Autodesk Fusion 360 part; units mm, degrees
sketch "Sketch1" plane through (0, 0, 0) normal (0, 0, 1) x (1, 0, 0)
  line L0 (0, 0) -> (-178, 0)
  line L1 (-178, 0) -> (-178, 64)
  line L2 (-178, 64) -> (0, 64)
  line L3 (0, 64) -> (0, 0)
  dimension "d1" = 64
  dimension "d2" = 178
extrude "Extrude1" add sketch "Sketch1" along normal blind 19
fillet "Fillet1" radius 32 4 edges at (0, 0, 9.5) (0, 64, 9.5) (-178, 0, 9.5) (-178, 64, 9.5)
sketch "Sketch2" plane through (0, 0, 19) normal (0, 0, 1) x (-1, 0, 0)
  arc A0 (146, -64) -> (146, 0) centre (146, -32) ccw
  line L0 (146, 0) -> (32, 0)
  arc A1 (32, 0) -> (32, -64) centre (32, -32) ccw
  line L1 (32, -64) -> (146, -64)
  line L2 (89, -64) -> (89, 0) construction
  circle A2 centre (32, -32) radius 10.5
  circle A3 centre (146, -32) radius 10.5
  dimension "d6" = 21
extrude "Extrude2" cut sketch "Sketch2" against normal blind 90 contours A2 | A3
sketch "Sketch3" plane through (0, 0, 19) normal (0, 0, 1) x (-1, 0, 0)
  circle A0 centre (32, -32) radius 10.5
  circle A1 centre (146, -32) radius 10.5
  arc A2 (146, -64) -> (146, 0) centre (146, -32) ccw
  line L0 (146, 0) -> (32, 0)
  arc A3 (32, 0) -> (32, -64) centre (32, -32) ccw
  line L1 (32, -64) -> (146, -64)
  line L2 (146, -64) -> (32, -64) construction
  line L3 (89, -64) -> (89, 0) construction
  line L4 (89, -64) -> (57, -64)
  line L5 (121, -64) -> (108, -64)
  line L6 (108, -64) -> (108, 0)
  line L7 (108, 0) -> (121, 0)
  line L8 (121, 0) -> (121, -64)
  line L9 (121, -64) -> (108, -64)
  line L10 (108, -64) -> (108, 0)
  line L11 (108, 0) -> (121, 0)
  line L12 (121, 0) -> (121, -64)
  line L13 (70, -64) -> (70, 0)
  line L14 (57, -64) -> (70, -64)
  line L15 (57, 0) -> (57, -64)
  line L16 (70, 0) -> (57, 0)
  line L17 (108, -64) -> (70, -64)
  line L18 (70, -64) -> (70, -51)
  line L19 (70, -51) -> (108, -51)
  line L20 (108, -51) -> (108, -64)
  dimension "d9" = 32
  dimension "d10" = 32
  dimension "d11" = 13
  dimension "d12" = 64
  dimension "d13" = 13
extrude "Extrude3" add sketch "Sketch3" along normal blind 45 contours L0 L1 L5 L6 L7 L8 L9 L10 L11 L12 L20 | L1 L4 L6 L10 L13 L17 L18 L19 L20 | L0 L1 L4 L13 L14 L15 L16 L18
sketch "Sketch4" plane through (-108, 0, 0) normal (1, 0, 0) x (0, 1, 0)
  line L0 (0, 19) -> (51, 19)
  line L1 (51, 19) -> (51, 64)
  line L2 (51, 64) -> (0, 64)
  line L3 (0, 64) -> (0, 19)
  line L4 (51, 64) -> (0, 19)
  line L5 (51, 19) -> (51, 64)
  line L6 (51, 19) -> (0, 19)
extrude "Extrude4" add sketch "Sketch4" along normal blind 38 contours L0 L1 L4 L5 L6
equation "d2 = 114 mm + 32 mm + 32 mm"
equation "d11 = ( ( 64 - 38 ) / 2 ) * 1 mm"
equation "d13 = 64 mm - 51 mm"
equation "d14 = 64 mm - 19 mm"
Input: part model. Units: mm. Frame: model coordinates. A direction names the side the tool comes from. Coordinates: 2 decimals unless noted, no trailing zeros. Loops run counter-clockwise (first coordinate to the right, second up) from the corner with the lowest first, then second, coordinate; pieces in that order, holes last. Notation, with made-up numbers: M 87,17.5 L 139,17.5 A13 cw 139,26.5 Z; hole C 19,38 d2. An arc over 180 degrees is marked long. Answer in a Markdown table with one row per item.
1. Section A-A, the plane y = 30. Output: boundary loops of the cut face in (x, z).
Response:
| item | result |
|---|---|
| outline | M -177.94,0 L -156.31,0 L -156.31,19 L -177.94,19 Z; M -135.69,0 L -42.31,0 L -42.31,19 L -57,19 L -57,64 L -70,64 L -70,45.47 L -108,45.47 L -108,64 L -121,64 L -121,19 L -135.69,19 Z; M -21.69,0 L -0.06,0 L -0.06,19 L -21.69,19 Z |
2. Section C-C, the plane x = -101.5. Output: boundary loops of the cut face in (y, z).
Response:
| item | result |
|---|---|
| outline | M 0,0 L 64,0 L 64,64 L 51,64 L 0,19 Z |
3. First-contact query: pin 1 (1 mm diameter, centred on x = -43, y = 25, fed in from +Z); pin 2 (1.5 mm diameter, centred on y = 45, z = 46.5, fed in from +X); pin 3 (4 mm diameter, centred on x = -79.5, z = 44, fed in from -Y); pin 4 (5 mm diameter, centred on x = -142, z = 23, fed in from +Y). Flat tips, straight axial feed; report the tip coordinate or a pass-through.
Response:
| item | result |
|---|---|
| pin 1 | stops at z = 19 |
| pin 2 | stops at x = -57 |
| pin 3 | stops at y = 26.07 |
| pin 4 | passes through |
4. Section B-B, the plane z = 6. Count the separate pieces of the cut face and the enclosed holes in it, then the cut area to 3 significant figures.
Response:
| item | result |
|---|---|
| separate pieces | 1 |
| enclosed holes | 2 |
| area | 9,820 mm2 |
5. Section D-D, the plane z = 56.5. Output: boundary loops of the cut face in (x, y), then the cut area to 3 significant figures.
Response:
| item | result |
|---|---|
| outline | M -121,0 L -108,0 L -108,42.5 L -70,42.5 L -70,0 L -57,0 L -57,64 L -121,64 Z |
| area | 2,480 mm2 |
6. Material intervals for line 1 (X direction, y = 32, z = 13.75); line 2 (Y direction, x = -32, z = 14.25); line 3 (X direction, y = 40, z = 7), sorted ascending.
Response:
| item | result |
|---|---|
| line 1 | x = -178 to -156.5, -135.5 to -42.5, -21.5 to 0 |
| line 2 | y = 0 to 21.5, 42.5 to 64 |
| line 3 | x = -176.99 to -152.8, -139.2 to -38.8, -25.2 to -1.01 |
7. Reachability of faces 1 (the flat face through (-156, 40, 19)), 2 (the flat face through (-57, 32, 41)), 3 (the cylindrical face through (-138.261, 24.904, 9.633)), 4 (the flat face through (-89.266, 25.857, 41.815)) from +Z, -Z, +X, -X, +Y, -Y: full face, straight path, thin tool, end or side. Return the list, or none.
Response:
| item | result |
|---|---|
| face 1 | +Z, -X, +Y, -Y |
| face 2 | +Z, +X, +Y, -Y |
| face 3 | +Z, -Z |
| face 4 | +Z, -Y |
8. Draft query along Y for faces 5 (the cylindrical face through (-24.261, 24.904, 9.633)), 6 (the flat face through (-121, 32, 41)), 7 (the cylindrical face through (-9.621, 9.123, 9.633)), 8 (the cylindrical face through (-168.379, 54.877, 9.633)). Return one class per face: pulls with the +Y half, pulls with the -Y half, needs draft (parallel to the pull), parting line crosses it, or undercut.
Response:
| item | result |
|---|---|
| face 5 | undercut |
| face 6 | needs draft |
| face 7 | pulls with the -Y half |
| face 8 | pulls with the +Y half |
